CAD build for the part. Positions are in the model's coordinates, mm. Face numbers are marked on the shaded views. Give positions to 0.01 mm unless a question says otherwise; leave off trailing zeros. Loops run counter-clockwise (first coordinate to the right, second up) from the corner with the lowest first, then second, coordinate; pieces in that order, holes last. Notation, with made-up numbers: (-29.5, 84.25) - (-20.5, 84.25) arc R27 ccw to (-20.5, 117.25) - close; hole circle Ø4 at (60.25, 77). An arc over 180 degrees is marked (long way). Return JSON: item names as keys, results as strings.
from build123d import *

# Parameters (mm, degrees)
SKETCH1_R           = 25
BOSS_EXTRUDE1_DEPTH = 2
SKETCH2_R           = 27
SKETCH2_R_2         = 25
BOSS_EXTRUDE2_DEPTH = 7
CUT_EXTRUDE1_DEPTH  = 49.590122453
CHAMFER1_SIZE       = 0.5


with BuildPart() as part:
    # Sketch1 → Boss-Extrude1 (new body)
    with BuildSketch(Plane.XY):
        with BuildLine():
            Line((-11.5, 30.659419425), (-11.5, 31.464265445))
            ThreePointArc((-11.5, 31.464265445), (-11.36006594, 31.900521733), (-10.992481203, 32.173985718))
            ThreePointArc((-10.992481203, 32.173985718), (0, 34), (10.992481203, 32.173985718))
            ThreePointArc((10.992481203, 32.173985718), (11.36006594, 31.900521733), (11.5, 31.464265445))
            Line((11.5, 31.464265445), (11.5, 30.659419425))
            ThreePointArc((11.5, 30.659419425), (11.824896973, 29.566702695), (12.694029851, 28.829006324))
            ThreePointArc((12.694029851, 28.829006324), (22.273863602, 22.273863602), (28.829006324, 12.694029851))
            ThreePointArc((28.829006324, 12.694029851), (29.566702695, 11.824896973), (30.659419425, 11.5))
            Line((30.659419425, 11.5), (31.464265445, 11.5))
            ThreePointArc((31.464265445, 11.5), (31.900521733, 11.36006594), (32.173985718, 10.992481203))
            ThreePointArc((32.173985718, 10.992481203), (34, 0), (32.173985718, -10.992481203))
            ThreePointArc((32.173985718, -10.992481203), (31.900521733, -11.36006594), (31.464265445, -11.5))
            Line((31.464265445, -11.5), (30.659419425, -11.5))
            ThreePointArc((30.659419425, -11.5), (29.566702695, -11.824896973), (28.829006324, -12.694029851))
            ThreePointArc((28.829006324, -12.694029851), (22.273863602, -22.273863602), (12.694029851, -28.829006324))
            ThreePointArc((12.694029851, -28.829006324), (11.824896973, -29.566702695), (11.5, -30.659419425))
            Line((11.5, -30.659419425), (11.5, -31.464265445))
            ThreePointArc((11.5, -31.464265445), (11.36006594, -31.900521733), (10.992481203, -32.173985718))
            ThreePointArc((10.992481203, -32.173985718), (0, -34), (-10.992481203, -32.173985718))
            ThreePointArc((-10.992481203, -32.173985718), (-11.36006594, -31.900521733), (-11.5, -31.464265445))
            Line((-11.5, -31.464265445), (-11.5, -30.659419425))
            ThreePointArc((-11.5, -30.659419425), (-11.824896973, -29.566702695), (-12.694029851, -28.829006324))
            ThreePointArc((-12.694029851, -28.829006324), (-22.273863602, -22.273863602), (-28.829006324, -12.694029851))
            ThreePointArc((-28.829006324, -12.694029851), (-29.566702695, -11.824896973), (-30.659419425, -11.5))
            Line((-30.659419425, -11.5), (-31.464265445, -11.5))
            ThreePointArc((-31.464265445, -11.5), (-31.900521733, -11.36006594), (-32.173985718, -10.992481203))
            ThreePointArc((-32.173985718, -10.992481203), (-34, 0), (-32.173985718, 10.992481203))
            ThreePointArc((-32.173985718, 10.992481203), (-31.900521733, 11.36006594), (-31.464265445, 11.5))
            Line((-31.464265445, 11.5), (-30.659419425, 11.5))
            ThreePointArc((-30.659419425, 11.5), (-29.566702695, 11.824896973), (-28.829006324, 12.694029851))
            ThreePointArc((-28.829006324, 12.694029851), (-22.273863602, 22.273863602), (-12.694029851, 28.829006324))
            ThreePointArc((-12.694029851, 28.829006324), (-11.824896973, 29.566702695), (-11.5, 30.659419425))
        make_face()
        Circle(SKETCH1_R, mode=Mode.SUBTRACT)
    extrude(amount=BOSS_EXTRUDE1_DEPTH)

    # Sketch2 → Boss-Extrude2 (add)
    with BuildSketch(Plane.XY.offset(2)):
        Circle(SKETCH2_R)
        Circle(SKETCH2_R_2, mode=Mode.SUBTRACT)
    extrude(amount=BOSS_EXTRUDE2_DEPTH)

    # Sketch3 → Cut-Extrude1 (cut, through all)
    with BuildSketch(Plane.XY.offset(2)):
        with BuildLine():
            Line((31.5, 1.5), (35.327471806, 1.5))
            Line((35.327471806, 1.5), (35.327471806, -1.5))
            Line((35.327471806, -1.5), (31.5, -1.5))
            ThreePointArc((31.5, -1.5), (30, 0), (31.5, 1.5))
        make_face()
        with BuildLine():
            Line((-1.5, -31.5), (-1.5, -34.385950358))
            Line((-1.5, -34.385950358), (1.5, -34.385950358))
            Line((1.5, -34.385950358), (1.5, -31.5))
            ThreePointArc((1.5, -31.5), (0, -30), (-1.5, -31.5))
        make_face()
        with BuildLine():
            Line((-31.5, -1.5), (-36.640801576, -1.5))
            Line((-36.640801576, -1.5), (-36.640801576, 1.5))
            Line((-36.640801576, 1.5), (-31.5, 1.5))
            ThreePointArc((-31.5, 1.5), (-30, 0), (-31.5, -1.5))
        make_face()
        with BuildLine():
            Line((-1.5, 31.5), (-1.5, 35.301296781))
            Line((-1.5, 35.301296781), (1.5, 35.301296781))
            Line((1.5, 35.301296781), (1.5, 31.5))
            ThreePointArc((1.5, 31.5), (0, 30), (-1.5, 31.5))
        make_face()
    extrude(amount=-CUT_EXTRUDE1_DEPTH, mode=Mode.SUBTRACT)

    # Chamfer1
    chamfer1_edges = [part.edges().sort_by_distance(p)[0] for p in [
        (-27, 0, 9),
    ]]
    chamfer(chamfer1_edges, length=CHAMFER1_SIZE)


solid = part.part
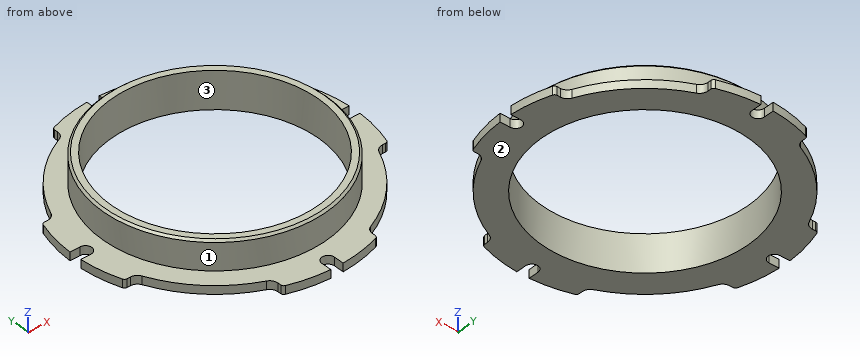
1. Drop flat-ended pins along their axis: P1, Ø3, axis at y = -19, z = 5, coming from the -X side; P2, Ø1.6, axis at x = 32.5, z = 0.5, coming from the -Y side; P3, Ø1, axis at y = -32, z = 1.5, coming from the +X side; P4, Ø12, axis at x = 8, y = -21.5, coming from the +Z side. Give the stop position or say it passes through.
Values follow:
{"P1": "stops at x = -20.56", "P2": "stops at y = -11.46", "P3": "stops at x = 11.5", "P4": "stops at z = 9"}
2. Cut at A-A, the plane z = 7.5. Write the cut outline in (x, y).
Values follow:
{"outline": "circle Ø54 at (0, 0); hole circle Ø50 at (0, 0)"}
3. Drill centre lines: probe 1 along Y at (x, z) = (0, 3); probe 2 along Y at (x, z) = (-8, 8.5); probe 3 along Z at (x, y) = (-15, -23.5). Where is each one in solid material? Low to high.
Values follow:
{"probe 1": "y = -27 to -25, 25 to 27", "probe 2": "y = -25.79 to -23.69, 23.69 to 25.79", "probe 3": "z = 0 to 2"}
4. Pull direction X, two halves, no side cores. Call the marked faces 1, 2 and 3: +X half, -X half, draft (parallel to the pull), parting line (faces both ways), or undercut.
Values follow:
{"face 1": "parting line", "face 2": "draft", "face 3": "undercut"}
